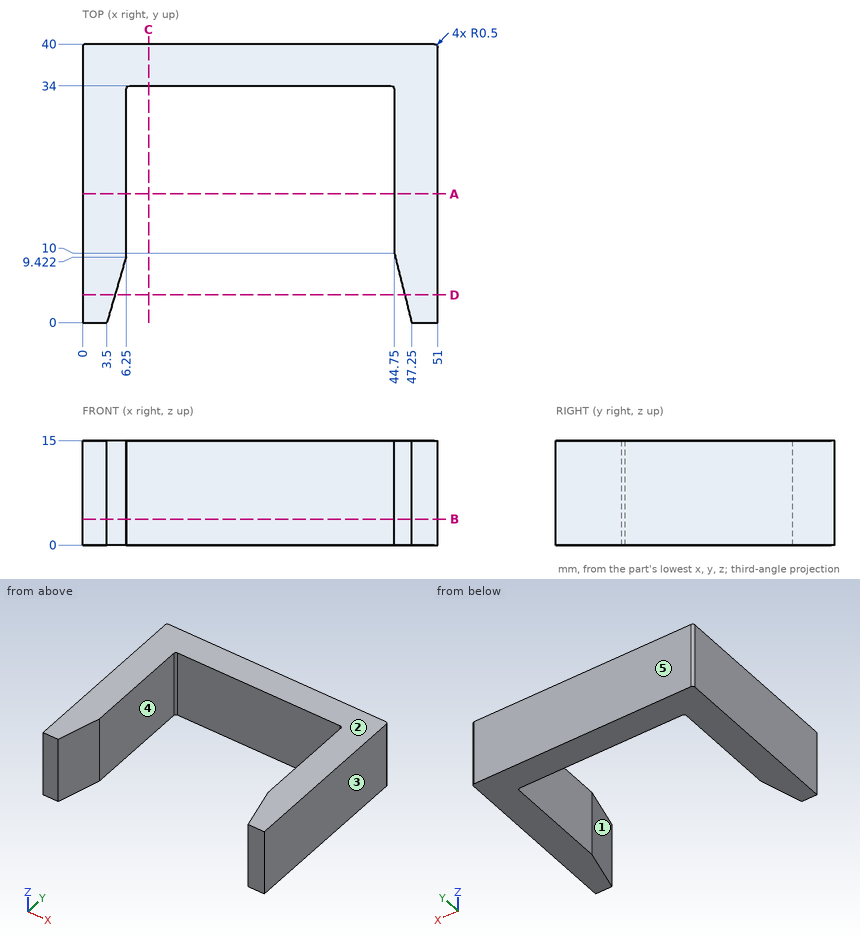
Geometry: see drawing. Coordinates: mm, zero at the bounding-box minimum. A direction names the side the tool comes from. Give positions to 0.01 mm unless a question says otherwise; leave off trailing zeros. Order: outer loops, then holes, each group sorted by start corner. A loop starts at its lowest first (then second) coordinate and runs counter-clockwise, first axis right, second up.
1. Cut plane A-A (y = 18.5). Return loops of the section in (x, z).
Computed:
outline: (0, 0) - (6.25, 0) - (6.25, 15) - (0, 15) - close; (44.75, 0) - (51, 0) - (51, 15) - (44.75, 15) - close
2. Cut plane C-C (x = 9.5). Return loops of the section in (y, z).
Computed:
outline: (34, 0) - (40, 0) - (40, 15) - (34, 15) - close
3. Line query: probe 1 along X at (y, z) = (16, 8); probe 2 along Y at (x, z) = (19.5, 1.25); probe 3 along X at (y, z) = (6.5, 8.75) (1 decimal). Output: solid intervals per line, ascending.
Computed:
probe 1: x = 0 to 6.25, 44.75 to 51
probe 2: y = 34 to 40
probe 3: x = 0 to 5.4, 45.6 to 51
4. Pin query (flat end, axial travel): pin 1 Ø2 at (x, y) = (19, 31.5) entering from -Z; pin 2 Ø6 at (x, z) = (35, 7) entering from -Y. Return the tip coordinate at first contact, or that it passes through.
Computed:
pin 1: passes through
pin 2: stops at y = 34
5. Set-up query: the marked faces 1 and 2. Return all of +Z, -Z, +X, -X, +Y, -Y with unobstructed straight access to the full face (end or side cutting, diameter ignored); none if empty.
Computed:
face 1: +Z, -Z, -Y
face 2: +Z, +X, -X, +Y, -Y
6. Cut plane D-D (y = 4). Return loops of the section in (x, z), and give its area (3 significant figures).
Computed:
outline: (0, 0) - (4.67, 0) - (4.67, 15) - (0, 15) - close; (46.25, 0) - (51, 0) - (51, 15) - (46.25, 15) - close
area: 141 mm2
7. Draft query along X for the marked faces 3, 4 and 5. Return one class per face: released by +X, released by -X, zero draft, split by the parting line, or undercut.
Computed:
face 3: released by +X
face 4: undercut
face 5: zero draft
8. Cut plane B-B (z = 3.75). Return loops of the section in (x, y).
Computed:
outline: (0, 0) - (3.5, 0) - (6.25, 9.42) - (6.25, 33.5) arc R0.5 cw to (6.75, 34) - (44.25, 34) arc R0.5 cw to (44.75, 33.5) - (44.75, 10) - (47.25, 0) - (51, 0) - (51, 39.5) arc R0.5 ccw to (50.5, 40) - (0.5, 40) arc R0.5 ccw to (0, 39.5) - close
